Input: part model. Units: mm. Frame: model coordinates. Face numbers are marked on the shaded views. A direction names the side the tool comes from. Coordinates: 2 decimals unless noted, no trailing zeros. Order: outer loops, then holes, each group sorted by start corner. A loop starts at its lowest first (then second) coordinate and runs counter-clockwise, first axis right, second up. Notation, with made-up numbers: (-15, 64.5) -> (10, 64.5) arc R26 ccw to (10, 79.5) -> close; hole circle Ø10 at (-8, -34.5). An arc over 180 degrees is marked (long way). Use CSV: the item, a comma, the result in double quotes. Start each with the question number.
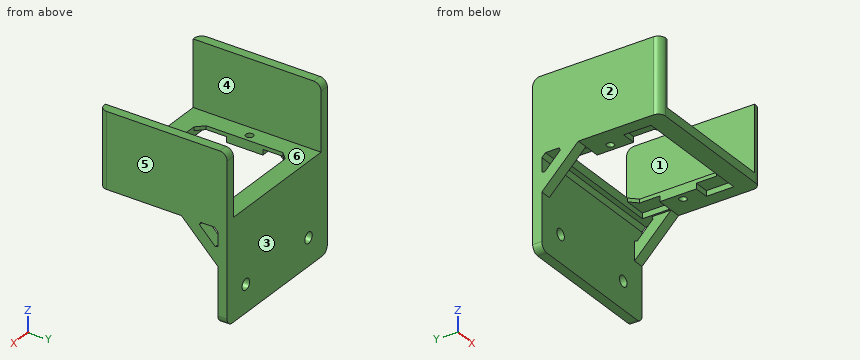
Autodesk Inventor part; units mm, degrees
ref_plane "Work Plane1" through (20, 2, 2.5) normal (1, 0, 0) x (0, 0, -1)
ref_plane "YZ Plane" through (0, 0, 0) normal (1, 0, 0) x (0, 1, 0)
ref_plane "XZ Plane" through (0, 0, 0) normal (0, 1, 0) x (-1, 0, 0)
sketch "Sketch1" plane through (0, 0, 0) normal (0, 0, 1) x (1, 0, 0)
  line L0 (0, 0) -> (40, 0)
  line L1 (40, 0) -> (40, 35)
  line L2 (40, 35) -> (0, 35)
  line L3 (0, 35) -> (0, 0)
  dimension "d0" = 35
  dimension "d1" = 40
extrude "Extrusion1" add sketch "Sketch1" along normal blind 2.5
sketch "Sketch2" plane through (0, 0, 2.5) normal (0, 0, 1) x (1, 0, 0)
  line L0 (7.5, 30) -> (32.5, 30)
  line L1 (32.5, 30) -> (32.5, 5)
  line L2 (32.5, 5) -> (7.5, 5)
  line L3 (7.5, 5) -> (7.5, 30)
  line L4 (0, 0) -> (40, 0)
  line L5 (0, 35) -> (0, 0)
  point P0 (20, 30)
  point P1 (20, 0)
  point P2 (7.5, 17.5)
  point P3 (0, 17.5)
  dimension "d4" = 25
extrude "Extrusion2" cut sketch "Sketch2" against normal through all
sketch "Sketch3" plane through (0, 0, 0) normal (0, 0, -1) x (-1, 0, 0)
  line L0 (-5.5, 17.5) -> (-34.5, 17.5)
  line L1 (0, 0) -> (-40, 0)
  line L2 (0, 35) -> (0, 0)
  point P0 (-20, 17.5)
  point P1 (-20, 0)
  point P2 (0, 17.5)
  dimension "d7" = 29
hole "Hole1" at (5.5, 17.5, 0) at (34.5, 17.5, 0) direction (0, 0, 1) diameter 2 end through all
sketch "Sketch4" plane through (0, 0, 0) normal (0, 0, -1) x (-1, 0, 0)
  line L0 (-40, 0) -> (-40, 35)
  line L1 (0, 35) -> (0, 0)
  line L2 (-40, 35) -> (0, 35)
  line L3 (0, 35) -> (0, 32.5)
  line L4 (0, 32.5) -> (-40, 32.5)
  line L5 (-40, 32.5) -> (-40, 35)
  dimension "d15" = 2.5
extrude "Extrusion3" add sketch "Sketch4" along normal blind 25
fillet "Fillet1" radius 2 4 edges at (40, 0, 1.25) (0, 0, 1.25) (0, 33.75, -25) (40, 33.75, -25)
chamfer "Chamfer1" distance 2 angle 45 4 edges at (7.5, 30, 1.25) (32.5, 30, 1.25) (32.5, 5, 1.25) (7.5, 5, 1.25)
sketch "Sketch5" plane through (40, 2, 0) normal (1, 0, 0) x (0, 0, -1)
  line L0 (0, 30.5) -> (23, 30.5)
  line L1 (10, 30.5) -> (0, 20.5)
  line L2 (0, 0) -> (0, 30.5)
  line L3 (7.8787, 32.6213) -> (-2.1213, 22.6213)
  point P0 (0, -2)
  point P1 (5.7574, 30.5)
  point P2 (0, 24.7426)
  dimension "d22" = 10
  dimension "d23" = 10
  dimension "d24" = 3
extrude "Extrusion4" add sketch "Sketch5" against normal blind 3 contours L0 L1 L2 L3
ref_plane "Work Plane1" through (20, 2, 2.5) normal (1, 0, 0) x (0, 0, -1)
mirror "Mirror1" about plane through (20, 2, 2.5) normal (1, 0, 0) of "Extrusion4"
sketch "Sketch6" plane through (0, 32.5, 0) normal (0, -1, 0) x (1, 0, 0)
  line L0 (7.5, -17.5) -> (32.5, -17.5)
  line L1 (38, -25) -> (2, -25)
  point P0 (0, 0)
  point P1 (20, -17.5)
  point P2 (20, -25)
  dimension "d27" = 25
  dimension "d28" = 7.5
hole "Hole2" at (7.5, 32.5, -17.5) at (32.5, 32.5, -17.5) direction (0, 1, 0) diameter 3 end through all
chamfer "Chamfer2" distance 1 angle 45 5 edges at (20, 32.5, 0) (1.5, 32.5, -5.7574) (1.5, 26.7426, 0) (38.5, 32.5, -5.7574) (38.5, 26.7426, 0)
sketch "Sketch7" plane through (0, 0, 0) normal (0, 0, -1) x (-1, 0, 0)
  line L0 (-30.5, 30) -> (-9.5, 30)
  line L1 (-30.5, 30) -> (-36.5, 30)
  line L2 (-36.5, 30) -> (-36.5, 5)
  line L3 (-36.5, 5) -> (-30.5, 5)
  line L4 (-32.5, 7) -> (-30.5, 5)
  line L5 (-32.5, 7) -> (-32.5, 28)
  line L6 (-30.5, 30) -> (-32.5, 28)
  line L7 (-32.5, 22.5) -> (-36.5, 22.5)
  line L8 (-32.5, 12.5) -> (-36.5, 12.5)
  line L9 (-34.5, 22.5) -> (-34.5, 12.5) construction
  point P0 (0, 0)
  point P1 (-34.5, 17.5)
  point P2 (-32.5, 17.5)
  dimension "d39" = 6
  dimension "d40" = 10
extrude "Extrusion5" cut sketch "Sketch7" against normal blind 1.5 contours L6 L5 L7 L2 L1 | L8 L5 L4 L3 L2
mirror "Mirror2" about plane through (20, 2, 2.5) normal (1, 0, 0) of "Extrusion5"
sketch "Sketch8" plane through (0, 0, 2.5) normal (0, 0, 1) x (1, 0, 0)
  line L0 (0, 35) -> (0, 2)
  arc A0 (0, 2) -> (2, 0) centre (2, 2) ccw
  line L1 (2, 0) -> (2.5, 0)
  line L2 (2, 0) -> (38, 0)
  line L3 (2.5, 0) -> (2.5, 35)
  line L4 (0, 32.5) -> (0, 35)
  line L5 (2.5, 35) -> (0, 35)
  point P0 (0, 0)
  dimension "d43" = 0.5
extrude "Extrusion6" add sketch "Sketch8" along normal blind 18
fillet "Fillet2" radius 2 1 edges at (1.25, 35, 20.5)
mirror "Mirror3" about plane through (20, 2, 2.5) normal (1, 0, 0) of "Extrusion6", "Fillet2"
properties part number "PIR mount"
1. Section D-D on x = 11. Return loops of the section in (y, z), then the cut area to 3 significant figures.
2. Material intervals for line 1 along X through (y, z) = (33.6, -17.5); line 2 along Y through (x, z) = (5.5, 0.85); line 3 along X through (y, z) = (17.5, 0.55), sorted ascending.
3. Contact query for flat-ended pins moving along their axis: P1, Ø12, axis at x = 10, y = 21.5, coming from the -Z side; P2, Ø3, axis at x = 6, y = 8, coming from the -Z side; P3, Ø6.5, axis at x = 5.5, y = 24.5, coming from the -Z side. Output: stop coordinate, or through.
4. Pull-direction query (X, two-part tool) for the marked faces 3, 4, 5 and 6; classes: released by +X, released by -X, zero draft, split by the parting line, or undercut.
5. Section A-A on y = 8. Return loops of the section in (x, z).
6. Section B-B on y = 17.5. Return loops of the section in (x, z).
7. Access query for the marked faces 1 and 2. Directions: +Z, -Z, +X, -X, +Y, -Y. A direction counts if a zero-diameter tool reaches every point of the face in a straight line with its end or side. Return the directions, or none.
8. Section C-C on z = 12. Return loops of the section in (x, y).
Values follow:
1,outline,"(0, 0) -> (5, 0) -> (5, 2.5) -> (0, 2.5) -> close; (30, 0) -> (31.5, 0) -> (32.5, -1) -> (32.5, -25) -> (35, -25) -> (35, 2.5) -> (30, 2.5) -> close"
1,area,"88.0 mm2"
2,line 1,"x = 0 to 6, 9 to 31, 34 to 40"
2,line 2,"y = 0 to 5, 12.5 to 16.5, 18.5 to 22.5, 30 to 35"
2,line 3,"x = 0 to 4.5, 6.5 to 7.5, 32.5 to 33.5, 35.5 to 40"
3,P1,"stops at z = 0"
3,P2,"stops at z = 1.5"
3,P3,"stops at z = -4.08"
4,face 3,"zero draft"
4,face 4,"undercut"
4,face 5,"released by +X"
4,face 6,"undercut"
5,outline,"(0, 0) -> (3.5, 0) -> (3.5, 1.5) -> (7.5, 1.5) -> (7.5, 2.5) -> (2.5, 2.5) -> (2.5, 20.5) -> (0, 20.5) -> close; (32.5, 1.5) -> (36.5, 1.5) -> (36.5, 0) -> (40, 0) -> (40, 20.5) -> (37.5, 20.5) -> (37.5, 2.5) -> (32.5, 2.5) -> close"
6,outline,"(0, 0) -> (4.5, 0) -> (4.5, 2.5) -> (2.5, 2.5) -> (2.5, 20.5) -> (0, 20.5) -> close; (6.5, 0) -> (7.5, 0) -> (7.5, 2.5) -> (6.5, 2.5) -> close; (32.5, 0) -> (33.5, 0) -> (33.5, 2.5) -> (32.5, 2.5) -> close; (35.5, 0) -> (40, 0) -> (40, 20.5) -> (37.5, 20.5) -> (37.5, 2.5) -> (35.5, 2.5) -> close"
7,face 1,"+Z, +Y, -Y"
7,face 2,"+Z, -Z, -X, +Y, -Y"
8,outline,"(0, 2) arc R2 ccw to (2, 0) -> (2.5, 0) -> (2.5, 35) -> (0, 35) -> close; (37.5, 0) -> (38, 0) arc R2 ccw to (40, 2) -> (40, 35) -> (37.5, 35) -> close"
